from build123d import *

# Parameters (mm, degrees)
SKETCH1_R             = 0.7
BOSS_EXTRUDE1_DEPTH   = 4.348
BOSS_EXTRUDE1_2_DEPTH = 4.348
SKETCH3_W             = 8
SKETCH3_H             = 2.9
BOSS_EXTRUDE2_DEPTH   = 1.598
BOSS_EXTRUDE3_DEPTH   = 2
MOVE_FACE1_BY         = 0.35
CHAMFER1_SIZE         = 0.5
BOSS_EXTRUDE4_DEPTH   = 2.9
MOVE_FACE2_DEPTH      = 2.9


# Read off the part's stored shape, not the designer's step: Move Face2
with BuildPart() as part:
    # Sketch1 → Boss-Extrude1 (new body)
    with BuildSketch(Plane(origin=(0, 0, 0), x_dir=(-0.8660254037844383, 0, 0.5000000000000009), z_dir=(-0.5000000000000008, 0, -0.8660254037844382))):
        Polygon((-11.354412945, 1.65), (-11.354412945, 2.9), (-16, 2.9), (-16, 0), (-11.354412945, 0), align=None)
        with Locations((-12.854412945, 1.575)):
            Circle(SKETCH1_R, mode=Mode.SUBTRACT)
    extrude(amount=BOSS_EXTRUDE1_DEPTH)



with BuildPart() as body_2:
    # Sketch1 → Boss-Extrude1 2 (new body)
    with BuildSketch(Plane(origin=(0, 0, 0), x_dir=(-0.8660254037844383, 0, 0.5000000000000009), z_dir=(-0.5000000000000008, 0, -0.8660254037844382))):
        Polygon((-3.354412945, 2.9), (-3.354412945, 1.65), (-3.354412945, 0), (0, 0), (0, 2.9), align=None)
        with Locations((-1.854412945, 1.575)):
            Circle(SKETCH1_R, mode=Mode.SUBTRACT)
    extrude(amount=BOSS_EXTRUDE1_2_DEPTH)


with BuildPart() as part_1:
    add(part.part)

    add(body_2.part)  # Boss-Extrude2 merges body 2
    # Sketch3 → Boss-Extrude2 (add)
    with BuildSketch(Plane(origin=(-2.174, 0, -3.765478456), x_dir=(-0.8660254037844384, 0, 0.5000000000000007), z_dir=(-0.5000000000000006, 0, -0.8660254037844383))):
        with Locations((-7.354412945, 1.45)):
            Rectangle(SKETCH3_W, SKETCH3_H)
    extrude(amount=-BOSS_EXTRUDE2_DEPTH)

    # Sketch4 → Boss-Extrude3 (add)
    with BuildSketch(Plane(origin=(-2.174, 0, -3.765478456), x_dir=(-0.8660254037844384, 0, 0.5000000000000007), z_dir=(-0.5000000000000006, 0, -0.8660254037844383))):
        Polygon((-1.214412945, 6.607188143), (-13.494412945, 6.607188143), (-13.494412945, 2.9), (-16, 2.9), (-16, 0), (0, 0), (0, 2.9), (-1.214412945, 2.9), align=None)
    extrude(amount=BOSS_EXTRUDE3_DEPTH)

    # Move Face1: a face moved inward by 0.35
    extrude(part_1.faces().sort_by_distance((-1.587, 1.45, -2.748764632))[0], amount=MOVE_FACE1_BY, dir=(0.866025404, 0, -0.5), mode=Mode.SUBTRACT)

    # Chamfer1
    chamfer1_edges = [part_1.edges().sort_by_distance(p)[0] for p in [
        (-1.622287539, 2.9, -5.238710332),
        (9.01250442, 2.9, -11.378710332),
    ]]
    chamfer(chamfer1_edges, length=CHAMFER1_SIZE)

    # Sketch5 → Boss-Extrude4 (add)
    with BuildSketch(Plane.XZ):
        with BuildLine():
            ThreePointArc((13.856406461, -8), (12.412098979, -10.837697405), (11.10213411, -13.739859135))
            Line((11.10213411, -13.739859135), (10.682406461, -13.497529263))
            Line((10.682406461, -13.497529263), (13.856406461, -8))
        make_face()
    extrude(amount=-BOSS_EXTRUDE4_DEPTH)

    # Move Face2 outline → Move Face2 (cut)
    with BuildSketch(Plane(origin=(0, 0, 0), x_dir=(1, 0, 0), z_dir=(0, 1, 0))):
        with BuildLine():
            ThreePointArc((10.97124357, 13.664289446), (12.281828843, 10.762456911), (13.726446616, 7.924967649))
            Line((13.726446616, 7.924967649), (13.856406461, 8))
            ThreePointArc((13.856406461, 8), (12.412098979, 10.837697405), (11.10213411, 13.739859135))
            Line((11.10213411, 13.739859135), (10.97124357, 13.664289446))
        make_face()
    extrude(amount=MOVE_FACE2_DEPTH, mode=Mode.SUBTRACT)


solid = part_1.part
The model under review builds one solid part; all positions refer to its coordinate system, in mm. A direction names the side the tool comes from. Round coordinates to 2 decimals unless told otherwise and drop trailing zeros. Write each loop counter-clockwise with the first axis right and the second up, starting at its lowest first coordinate (ties: lowest second). Pieces come first, ordered by that corner, then holes. Notation, with made-up numbers: M 73.5,62.25 L 127.5,62.25 A31 cw 127.5,96.25 Z; hole C 8,45.5 d4. An arc over 180 degrees is marked long. Use a Markdown table: item, result. Add a question column.
Q1. The part is to be moulded in two halves that separate along X. For faces 5 (the face through (9.24, 3.15, -11.49)), 6 (the face through (5, 0, -7)), 7 (the face through (5.043, 1.47, -6.087)), say which applies: pulls with the +X half, pulls with the -X half, needs draft (parallel to the pull), parting line crosses it, or undercut.
Q2. To check wall thickness, follow line 1 (Z direction, x = 2.75, y = 2.25); line 2 (X direction, y = 2, z = -3.5); line 3 (X direction, y = 0.75, z = -5.75). State the ranges of each line that lie inside material, in increasing order.
Q3. We need section C-C, the plane x = 5.25. State the section outline as (y, z) points, plus the area to 3 significant figures.
Q4. Insertion check: pin 1 (3 mm diameter, centred on x = 4.5, z = -4, fed in from +Y); pin 2 (1 mm diameter, centred on x = 1.5, y = 3, fed in from -Z); pin 3 (1.5 mm diameter, centred on x = 10, y = 1.5, fed in from +Z); pin 4 (3 mm diameter, centred on y = 3.5, z = -8, fed in from -X). Each pin has a flat end and moves straight along its axis. Give the tip position at first contact, or say it passes through.
Q5. We need section B-B, the plane z = -11.75. State the section outline as (x, y) points, plus the area to 3 significant figures.
Q6. We need section D-D, the plane y = 6. State the section outline as (x, z) points.
Q7. Machinability: for faces 1 (the face through (-0.56, 1.585, -4.698)), 2 (the face through (9, 5, -11.4)), 3 (the face through (4.28, 4.78, -7.49)), 4 (the face through (2.2, 1.5, -2.9)), which of the approach directions +Z, -Z, +X, -X, +Y, -Y give a long, thin tool a straight path to every point of the face, cutting with its end or side? Answer none if there is none.
Q8. We need section A-A, the plane y = 0.5. State the section outline as (x, z) points (3 decimals), plus the area to 3 significant figures.
Findings below:
| question | item | result |
|---|---|---|
| 1 | face 5 | pulls with the +X half |
| 1 | face 6 | needs draft |
| 1 | face 7 | undercut |
| 2 | line 1 | z = -8.92 to -4.76, -1.95 to -1.59 |
| 2 | line 2 | x = -1.62 to -0.52, 0.76 to 1.85 |
| 2 | line 3 | x = -2.74 to 4.46, 9.79 to 9.96 |
| 3 | outline | M 0,-10.36 L 6.61,-10.36 L 6.61,-8.05 L 2.9,-8.05 L 2.9,-6.21 L 0,-6.21 Z |
| 3 | area | 20.6 mm² |
| 4 | pin 1 | passes through |
| 4 | pin 2 | stops at z = -8.48 |
| 4 | pin 3 | stops at z = -5.68 |
| 4 | pin 4 | stops at x = -1.44 |
| 5 | outline | M 7.66,0 L 11.82,0 L 11.82,2.9 L 9.38,2.9 L 8.8,3.4 L 8.8,6.61 L 7.66,6.61 Z |
| 5 | area | 16.4 mm² |
| 6 | outline | M -2.12,-6.1 L 8.51,-12.24 L 9.51,-10.51 L -1.12,-4.37 Z |
| 7 | face 1 | none |
| 7 | face 2 | -Z, +X, +Y |
| 7 | face 3 | +Z, +X, +Y |
| 7 | face 4 | +X, +Y, -Y |
| 8 | outline | M -2.871,-5.673 L 10.971,-13.664 A68.19 cw 13.726,-7.925 L 9.833,-5.677 L 8.458,-8.059 L 1.53,-4.059 L 2.905,-1.677 L 0.303,-0.175 Z |
| 8 | area | 77.6 mm² |
